```python
from build123d import *

# Parameters (mm, degrees)
F0_R         = 6
F1_DEPTH     = 6
F2_W         = 7.68
F2_H         = 5.1
F3_DEPTH     = 25
F4_R         = 2.4142135624
F5_SIZE2     = 0.5
F5_SIZE      = 4.5
F6_T1_DEPTH  = 2.8515728753
F6_T3_DEPTH  = 0.2715728753
F6_T6_ANGLE  = 90
F6_T8_ANGLE  = 90
F6_T10_ANGLE = 90
F6_T12_ANGLE = 90


# Not quite as in the source:
# - a fillet or chamfer that OpenCascade refuses, or shapes differently, is made with other operations: its cross-section is extruded or revolved along the edge and cut away or added


with BuildPart() as f1:
    # F0 (on Top) → F1 (new body)
    with BuildSketch(Plane.XY):
        Circle(F0_R)
    extrude(amount=F1_DEPTH)

    # F2 (on face) → F3 (cut)
    with BuildSketch(Plane.XY.offset(6)):
        with Locations((0, -1.3597839279)):
            Rectangle(F2_W, F2_H)
    extrude(amount=-F3_DEPTH, mode=Mode.SUBTRACT)

    # F4
    f4_edges = [f1.edges().sort_by_distance(p)[0] for p in [
        (-3.84, 1.190216, 3),
        (3.84, 1.190216, 3),
        (3.84, -3.909784, 3),
        (-3.84, -3.909784, 3),
    ]]
    fillet(f4_edges, radius=F4_R)

    # F5
    f5_edges = [f1.edges().sort_by_distance(p)[0] for p in [
        (-6, 0, 0),
    ]]
    f5_side = f1.faces().sort_by_distance((-6, 0, 3))[0]
    chamfer(f5_edges, length=F5_SIZE, length2=F5_SIZE2, reference=f5_side)

    # F6: fillet of radius 1.2795331881 on 8 edges, made by hand

    # F6_s2 → F6_t1 (cut)
    with BuildSketch(Plane.YZ.offset(-1.4257864376)):
        with BuildLine():
            ThreePointArc((-5.189317116, 0), (-4.2845505219, 0.374766594), (-3.9097839279, 1.2795331881))
            Line((-3.9097839279, 1.2795331881), (-3.9097839279, 0))
            Line((-3.9097839279, 0), (-5.189317116, 0))
        make_face()
        with BuildLine():
            ThreePointArc((2.4697492601, 0), (1.5649826661, 0.374766594), (1.1902160721, 1.2795331881))
            Line((1.1902160721, 1.2795331881), (1.1902160721, 0))
            Line((1.1902160721, 0), (2.4697492601, 0))
        make_face()
    extrude(amount=F6_T1_DEPTH, mode=Mode.SUBTRACT)

    # F6_s4 → F6_t3 (cut)
    with BuildSketch(Plane.XZ.offset(1.2239974903)):
        with BuildLine():
            ThreePointArc((-5.1195331881, 0), (-4.214766594, 0.374766594), (-3.84, 1.2795331881))
            Line((-3.84, 1.2795331881), (-3.84, 0))
            Line((-3.84, 0), (-5.1195331881, 0))
        make_face()
        with BuildLine():
            ThreePointArc((5.1195331881, 0), (4.214766594, 0.374766594), (3.84, 1.2795331881))
            Line((3.84, 1.2795331881), (3.84, 0))
            Line((3.84, 0), (5.1195331881, 0))
        make_face()
    extrude(amount=F6_T3_DEPTH, mode=Mode.SUBTRACT)

    # F6_s5 → F6_t6 (revolve, cut)
    with BuildSketch(Plane.YZ.offset(-1.4257864376)):
        with BuildLine():
            ThreePointArc((2.4697492601, 0), (1.5649826661, 0.374766594), (1.1902160721, 1.2795331881))
            Line((1.1902160721, 1.2795331881), (1.1902160721, 0))
            Line((1.1902160721, 0), (2.4697492601, 0))
        make_face()
    revolve(axis=Axis((-1.4257864376, -1.2239974903, 0), (0, 0, 1)), revolution_arc=F6_T6_ANGLE, mode=Mode.SUBTRACT)

    # F6_s7 → F6_t8 (revolve, cut)
    with BuildSketch(Plane.YZ.offset(-1.4257864376)):
        with BuildLine():
            ThreePointArc((-5.189317116, 0), (-4.2845505219, 0.374766594), (-3.9097839279, 1.2795331881))
            Line((-3.9097839279, 1.2795331881), (-3.9097839279, 0))
            Line((-3.9097839279, 0), (-5.189317116, 0))
        make_face()
    revolve(axis=Axis((-1.4257864376, -1.4955703655, 0), (0, 0, -1)), revolution_arc=F6_T8_ANGLE, mode=Mode.SUBTRACT)

    # F6_s9 → F6_t10 (revolve, cut)
    with BuildSketch(Plane.YZ.offset(1.4257864376)):
        with BuildLine():
            ThreePointArc((-5.189317116, 0), (-4.2845505219, 0.374766594), (-3.9097839279, 1.2795331881))
            Line((-3.9097839279, 1.2795331881), (-3.9097839279, 0))
            Line((-3.9097839279, 0), (-5.189317116, 0))
        make_face()
    revolve(axis=Axis((1.4257864376, -1.4955703655, 0), (0, 0, 1)), revolution_arc=F6_T10_ANGLE, mode=Mode.SUBTRACT)

    # F6_s11 → F6_t12 (revolve, cut)
    with BuildSketch(Plane.XZ.offset(1.2239974903)):
        with BuildLine():
            ThreePointArc((5.1195331881, 0), (4.214766594, 0.374766594), (3.84, 1.2795331881))
            Line((3.84, 1.2795331881), (3.84, 0))
            Line((3.84, 0), (5.1195331881, 0))
        make_face()
    revolve(axis=Axis((1.4257864376, -1.2239974903, 0), (0, 0, 1)), revolution_arc=F6_T12_ANGLE, mode=Mode.SUBTRACT)


solid = f1.part
```
For this review, take the finished solid that the model builds, in its own axes (mm). A direction names the side the tool comes from. Give positions to 0.01 mm unless a question says otherwise; leave off trailing zeros. Loops run counter-clockwise (first coordinate to the right, second up) from the corner with the lowest first, then second, coordinate; pieces in that order, holes last. Notation, with made-up numbers: M -27,73 L -14,73 A24 ccw -14,94 Z; hole C 76.5,18 d2. An arc over 180 degrees is marked long. One line per item, written item: value. Start each with the question number.
Q1. Add section B-B (x = 0). Give the boundary of the cut face in (y, z).
Q2. Draft analysis for pull direction X (two halves, no side actions). For faces 4 (the face through (-6, 0, 5)), 5 (the face through (-0.02, -4.295, 0.365)), 6 (the face through (-0.1, 1.4, 6)), state which applies: released by +X, released by -X, zero draft, split by the parting line, or undercut.
Q3. Clearance check with flat-ended pins moving along their axes: pin 1 Ø2 at (x, z) = (2.5, 3) entering from -Y; pin 2 Ø3 at (x, z) = (0, 2.5) entering from -Y; pin 3 Ø2 at (x, z) = (-2.5, 1) entering from -Y. State where each tip first meets the part, or that it passes through.
Q4. For L1, parallel to Y at x = 0, z = 5; L2, parallel to Y at x = -3.5, z = 1.25; L3, parallel to X at y = 0, z = 2.5, list the stretches that pass through material, from the lowest coordinate up.
Q5. Machinability: for faces 1 (the face through (0, 3, 0)), 2 (the face through (0, -3.91, 4)), 3 (the face through (-0.02, 1.575, 0.365)), which of the approach directions +Z, -Z, +X, -X, +Y, -Y give a long, thin tool a straight path to every point of the face, cutting with its end or side? Answer none if there is none.
Q6. Add section A-A (z = 4.75). Give the boundary of the cut face in (x, y).
Q7. Add section C-C (z = 2). Give the boundary of the cut face in (x, y).
Reply:
1. outline: M -6,4.5 L -5.5,0 L -5.19,0 A1.28 ccw -3.91,1.28 L -3.91,6 L -6,6 Z; M 1.19,1.28 A1.28 ccw 2.47,0 L 5.5,0 L 6,4.5 L 6,6 L 1.19,6 Z
2. face 4: split by the parting line
2. face 5: undercut
2. face 6: zero draft
3. pin 1: y = -5.66
3. pin 2: y = -5.94
3. pin 3: y = -5.43
4. L1: -6 to -3.91, 1.19 to 6
4. L2: -4.42 to -2.73, 0.01 to 4.42
4. L3: -5.78 to -3.51, 3.51 to 5.78
5. face 1: -Z, +X, -X, +Y, -Y
5. face 2: +Z, -Z
5. face 3: -Z
6. outline: C 0,0 d12; hole M -3.84,-1.5 A2.41 ccw -1.43,-3.91 L 1.43,-3.91 A2.41 ccw 3.84,-1.5 L 3.84,-1.22 A2.41 ccw 1.43,1.19 L -1.43,1.19 A2.41 ccw -3.84,-1.22 Z
7. outline: C 0,0 d11.44; hole M -3.84,-1.5 A2.41 ccw -1.43,-3.91 L 1.43,-3.91 A2.41 ccw 3.84,-1.5 L 3.84,-1.22 A2.41 ccw 1.43,1.19 L -1.43,1.19 A2.41 ccw -3.84,-1.22 Z
